The listing builds one solid part. Answer for the finished solid, in the listing's coordinates (mm). Give positions to 0.01 mm unless a question says otherwise; leave off trailing zeros. Return JSON: item names as keys, results as strings.
Autodesk Inventor part; units mm, degrees
ref_plane "YZ Plane" through (0, 0, 0) normal (1, 0, 0) x (0, 1, 0)
ref_plane "XZ Plane" through (0, 0, 0) normal (0, 1, 0) x (-1, 0, 0)
ref_plane "XY Plane" through (0, 0, 0) normal (0, 0, 1) x (1, 0, 0)
ref_plane "Arbeitsebene1" through (0, -3.9, 0.8) normal (0, -1, 0) x (-1, 0, 0)
ref_plane "Arbeitsebene2" through (0, 0, 0) normal (0, 0, 1) x (1, 0, 0)
sketch "Skizze2" plane through (0, 0, 0) normal (0, 0, 1) x (1, 0, 0)
  circle A0 centre (31.3386, -4.2236) radius 0.75
  circle A1 centre (-0.1614, -4.2236) radius 0.75
  circle A2 centre (-31.3614, -4.2236) radius 0.75
  circle A3 centre (-32.5696, 4.2222) radius 0.75
  circle A4 centre (-0.1614, 4.2222) radius 0.75
  circle A5 centre (32.3386, 4.2222) radius 0.75
  circle A6 centre (36.7419, -1.8509) radius 0.75
  circle A7 centre (-36.6614, -1.7266) radius 0.75
  circle A8 centre (-36.6614, 1.7763) radius 0.75
  line L0 (33.8386, 4.2222) -> (-46.1614, 4.2222) construction
  line L1 (-46.1614, 4.2222) -> (-46.1614, -4.2236) construction
  line L2 (-46.1614, -4.2236) -> (33.8386, -4.2236) construction
  line L3 (33.8386, -4.2236) -> (33.8386, 4.2222) construction
  line L4 (33.8386, -4.2236) -> (36.7419, -4.2236) construction
  line L5 (36.7419, -4.2236) -> (36.7419, 4.2222) construction
  line L6 (36.7419, 4.2222) -> (33.8386, 4.2222) construction
  line L7 (33.8386, 4.2222) -> (33.8386, -4.2236) construction
  line L8 (-46.1614, -4.2236) -> (-36.6614, -4.2236) construction
  line L9 (-36.6614, -4.2236) -> (-36.6614, 4.2222) construction
  line L10 (-36.6614, 4.2222) -> (-46.1614, 4.2222) construction
  line L11 (-46.1614, 4.2222) -> (-46.1614, -4.2236) construction
  line L12 (38.2419, -5.2236) -> (-38.7581, -5.2236)
  line L13 (-38.7581, -5.2236) -> (-38.7581, 19.7764)
  line L14 (-38.7581, 19.7764) -> (38.2419, 19.7764)
  line L15 (38.2419, 19.7764) -> (38.2419, -5.2236)
  point P0 (0, 0)
  dimension "d0" = 1.5
  dimension "d1" = 8.4458
  dimension "d2" = 80
  dimension "d3" = 33.8386
  dimension "d4" = 4.2222
  dimension "d5" = 2.5
  dimension "d6" = 1.5
  dimension "d7" = 13.5918
  dimension "d8" = 14.8
  dimension "d9" = 34
  dimension "d10" = 34
  dimension "d11" = 2.9033
  dimension "d12" = 2.3726
  dimension "d13" = 9.5
  dimension "d14" = 2.497
  dimension "d15" = 2.4459
  dimension "d16" = 25
  dimension "d17" = 77
  dimension "d18" = 1.5
  dimension "d19" = 1
extrude "Extrusion1" add sketch "Skizze2" along normal blind 1.5
properties part number "Poti_Sensor_PCB_"
Item 1: Consider L1, parallel to X at y = 1.75, z = 0.6; L2, parallel to Y at x = -31.5, z = 0.7; L3, parallel to X at y = -1.25, z = 0.3. Determine where each line is inside the solid, lowest interval first.
Answer below:
{"L1": "x = -38.76 to -37.41, -35.91 to 38.24", "L2": "y = -5.22 to -4.96, -3.49 to 19.78", "L3": "x = -38.76 to -37.24, -36.08 to 36.29, 37.19 to 38.24"}
Item 2: Flat-ended cylindrical pins translate along their axes: P1, Ø0.9, axis at x = -31.36, y = -4.22, coming from the -Z side; P2, Ø2, axis at x = 31.34, y = -4.22, coming from the -Z side. Find the tip coordinate at first contact, or state that the pin passes through.
Answer below:
{"P1": "passes through", "P2": "stops at z = 0"}
Item 3: The mould has two halves that part along X. Classify faces 1 (the face through (-1, 19.776, 1)), 2 (the face through (32.031, -3.936, 0.74)), 3 (the face through (38.242, 7, 1)): +X half, -X half, draft (parallel to the pull), parting line (faces both ways), or undercut.
Answer below:
{"face 1": "draft", "face 2": "undercut", "face 3": "+X half"}
